from build123d import *

# Parameters (mm, degrees)
F1_DEPTH = 27.94
F2_R     = 2.428282
F2_R_2   = 2.464218
F3_DEPTH = 5.08
F4_W     = 5.207
F4_H     = 31.709664
F4_H_2   = 31.473025
F5_DEPTH = 23.622


with BuildPart() as f1:
    # F0 (on Right) → F1 (new body)
    with BuildSketch(Plane.YZ):
        with BuildLine():
            Line((-33.215124, 0), (-10.148687, 0))
            ThreePointArc((-10.148687, 0), (-3.800376, 2.735055), (0, 8.509024))
            ThreePointArc((0, 8.509024), (-4.54194, 4.408232), (-10.190163, 2.053812))
            Line((-10.190163, 2.053812), (-31.077091, 2.053812))
            Line((-31.077091, 2.053812), (-31.077091, 20.227084))
            Line((-31.077091, 20.227084), (-33.215124, 20.227084))
            Line((-33.215124, 20.227084), (-33.215124, 0))
        make_face()
    extrude(amount=F1_DEPTH)

    # F2 (on face) → F3 (cut)
    with BuildSketch(Plane(origin=(0, -31.077091, 0), x_dir=(-1, 0, 0), z_dir=(0, 1, 0))):
        with Locations((-5.342463, 9.339899)):
            Circle(F2_R)
        with Locations((-21.111647, 9.339899)):
            Circle(F2_R_2)
    extrude(amount=-F3_DEPTH, mode=Mode.SUBTRACT)

    # F4 (on Top) → F5 (cut)
    with BuildSketch(Plane.XY):
        with Locations((8.3185, -15.854832)):
            Rectangle(F4_W, F4_H)
        with Locations((19.6215, -15.736512)):
            Rectangle(F4_W, F4_H_2)
    extrude(amount=F5_DEPTH, mode=Mode.SUBTRACT)


solid = f1.part
Design review of the part built by this model. Coordinates are the model's own, in mm. A direction names the side the tool comes from. Round coordinates to 2 decimals unless told otherwise and drop trailing zeros. Write each loop counter-clockwise with the first axis right and the second up, starting at its lowest first coordinate (ties: lowest second). Pieces come first, ordered by that corner, then holes. Notation, with made-up numbers: (-22.5, 53) - (-9.5, 53) arc R33 cw to (-9.5, 81) - close; hole circle Ø2 at (12, 45). An arc over 180 degrees is marked (long way). Use a Markdown table: item, result. Add a question column.
1. Mouldability with a two-part tool opening along X and no side actions: class faces 1 (the face through (5.715, -17.1, 1.7)), 2 (the face through (27.94, -21.6, 1.9)), 3 (the face through (3, -31.077, 11)) as +X half, -X half, draft (parallel to the pull), parting line (faces both ways), or undercut.
2. Clearance check with flat-ended pins moving along their axes: pin 1 (9.5 mm diameter, centred on y = -23, z = 6, fed in from -X); pin 2 (1.7 mm diameter, centred on x = 26, y = -25.5, fed in from +Z); pin 3 (1.7 mm diameter, centred on x = 24, z = 11.5, fed in from +Y); pin 4 (4.5 mm diameter, centred on x = 21.11, z = 9.34, fed in from -Y). State where each tip first meets the part, or that it passes through.
3. Wall thickness on probe 1 along X at (y, z) = (-6, 3.25) (3 decimals); probe 2 along Y at (x, z) = (11.25, 17.25); probe 3 along Y at (x, z) = (22.5, 6): over which ranges is each line inside the solid? List them lowest first.
4. We need section D-D (z = 12.75). State the section outline as (x, y) points (3 decimals).
5. We need section A-A (y = -28). State the section outline as (x, z) points (3 decimals).
6. For faces 4 (the face through (23.573, -32.369, 9.448)), 5 (the face through (25.042, -4.469, 4.454)), 6 (the face through (17.018, -17, 1.8)), 7 (the face through (2.82, -3.88, 2.67)), 8 (the face through (14, -22, 0)), list the 3-axis set-ups (+Z, -Z, +X, -X, +Y, -Y) from which the entire face can be reached by the end or side of a thin tool; tool diameter is ignored.
7. We need section C-C (z = 10). State the section outline as (x, y) points.
8. We need section B-B (x = 21). State the section outline as (y, z) points.
Output:
| question | item | result |
|---|---|---|
| 1 | face 1 | undercut |
| 1 | face 2 | +X half |
| 1 | face 3 | draft |
| 2 | pin 1 | stops at x = 0 |
| 2 | pin 2 | stops at z = 2.05 |
| 2 | pin 3 | stops at y = -31.08 |
| 2 | pin 4 | stops at y = -0.96 |
| 3 | probe 1 | x = 0 to 5.715, 10.922 to 17.018, 22.225 to 27.94 |
| 3 | probe 2 | y = -33.22 to -31.08 |
| 3 | probe 3 | y = -33.22 to -31.08, -2.4 to -1.07 |
| 4 | outline | (0, -33.215) - (27.94, -33.215) - (27.94, -31.077) - (22.225, -31.077) - (22.225, -31.473) - (17.018, -31.473) - (17.018, -31.077) - (10.922, -31.077) - (10.922, -31.71) - (5.715, -31.71) - (5.715, -31.077) - (0, -31.077) - close |
| 5 | outline | (0, 0) - (5.715, 0) - (5.715, 2.054) - (0, 2.054) - close; (10.922, 0) - (17.018, 0) - (17.018, 2.054) - (10.922, 2.054) - close; (22.225, 0) - (27.94, 0) - (27.94, 2.054) - (22.225, 2.054) - close |
| 6 | face 4 | -Y |
| 6 | face 5 | +Z, +X, -X |
| 6 | face 6 | +Z, -Z, +Y |
| 6 | face 7 | -Z, +X, -X, +Y |
| 6 | face 8 | -Z, +X, -X, +Y, -Y |
| 7 | outline | (0, -33.22) - (3.01, -33.22) - (3.01, -31.08) - (0, -31.08) - close; (7.68, -33.22) - (18.74, -33.22) - (18.74, -31.47) - (17.02, -31.47) - (17.02, -31.08) - (10.92, -31.08) - (10.92, -31.71) - (7.68, -31.71) - close; (23.49, -33.22) - (27.94, -33.22) - (27.94, -31.08) - (23.49, -31.08) - close |
| 8 | outline | (-33.22, 0) - (-31.47, 0) - (-31.47, 6.88) - (-33.22, 6.88) - close; (-33.22, 11.8) - (-31.47, 11.8) - (-31.47, 20.23) - (-33.22, 20.23) - close |
